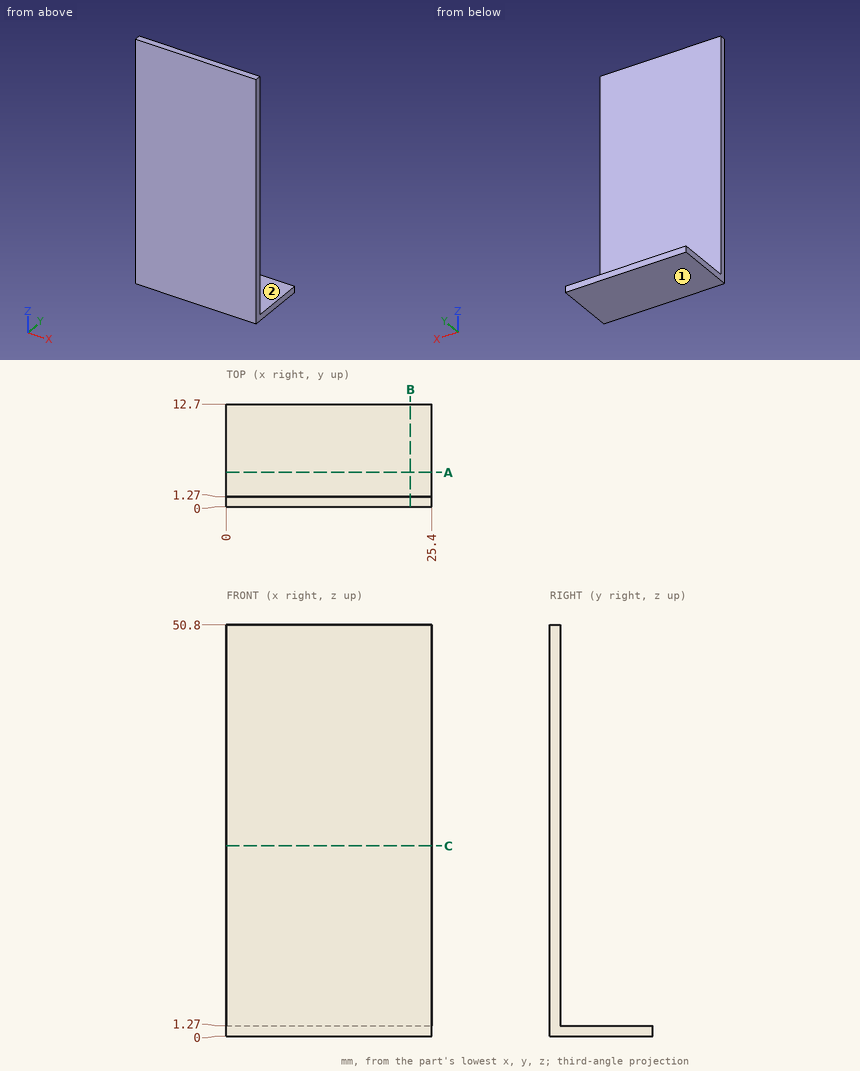
Print and shaded views of the part. All mm, measured from the part's lowest x, y and z. A direction names the side the tool comes from. Coordinates: 2 decimals unless noted, no trailing zeros. Loops run counter-clockwise (first coordinate to the right, second up) from the corner with the lowest first, then second, coordinate; pieces in that order, holes last. Notation, with made-up numbers: (57.5, 65) -> (94.5, 65) arc R27 ccw to (94.5, 101) -> close; hole circle Ø1 at (9.5, 80). An arc over 180 degrees is marked (long way). Use a Markdown table: item, result. Add a question column.
Item 1: Band-saw the part on A-A on y = 4.25. Write the cut outline in (x, z).
Item 2: Flat gauge pins, fed straight in: P1, Ø1.5, axis at x = 17.5, y = 9, coming from the +Z side; P2, Ø7.5, axis at x = 7.5, z = 25, coming from the +Y side. Where does each tip first touch, or does it go through?
Item 3: Band-saw the part on B-B on x = 22.75. Write the cut outline in (y, z).
Item 4: Probe probe 1 along Z at (x, y) = (4.5, 3.25). List the from-to ranges inside material, lowest first.
Item 5: Which spindle directions (+Z, -Z, +X, -X, +Y, -Y) get a long thin tool onto all of the face, cutting with end or side? Do the marked faces 1 and 2. Say none if no direction does.
Geometry says:
| question | item | result |
|---|---|---|
| 1 | outline | (0, 0) -> (25.4, 0) -> (25.4, 1.27) -> (0, 1.27) -> close |
| 2 | P1 | z = 1.27 |
| 2 | P2 | y = 1.27 |
| 3 | outline | (0, 0) -> (12.7, 0) -> (12.7, 1.27) -> (1.27, 1.27) -> (1.27, 50.8) -> (0, 50.8) -> close |
| 4 | probe 1 | 0 to 1.27 |
| 5 | face 1 | -Z, +X, -X, +Y, -Y |
| 5 | face 2 | +Z, +X, -X, +Y |
